The model under review builds one solid part; all positions refer to its coordinate system, in mm. Round coordinates to 2 decimals unless told otherwise and drop trailing zeros. Order: outer loops, then holes, each group sorted by start corner. A loop starts at its lowest first (then second) coordinate and runs counter-clockwise, first axis right, second up.
1) Consider section C-C (y = 0.2). Give the number of separate pieces and of enclosed holes in the cut face, then the cut area to 3 significant figures.
2) Consider section B-B (x = 0). Give the boundary of the cut face in (y, z), then the cut area to 4 significant figures.
3) Consider section D-D (z = 1). Give the boundary of the cut face in (x, y).
4) Consider section A-A (x = 5.1). Give the boundary of the cut face in (y, z).
5) To check wall thickness, follow L1, parallel to X at y = 0.1, z = 5.5; L2, parallel to Z at x = -2.3, y = 0.15; L3, parallel to X at y = 0.25, z = 1.25. State the ranges of each line that lie inside material, in increasing order.
from build123d import *

# Parameters (mm, degrees)
EXTRUDE1_DEPTH = 0.3
SKETCH3_R      = 0.4
SKETCH3_W      = 3
SKETCH3_H      = 1.2
EXTRUDE2_DEPTH = 1.3
SKETCH4_W      = 1
SKETCH4_H      = 0.25
EXTRUDE3_DEPTH = 24
SKETCH5_W      = 1.5
SKETCH5_H      = 1.5
EXTRUDE5_DEPTH = 1


with BuildPart() as part:
    # Sketch1 → Extrude1 (new body)
    with BuildSketch(Plane(origin=(0, 0, 0), x_dir=(1, 0, 0), z_dir=(0, 1, 0))):
        with BuildLine():
            Line((-2.435487214, 9.089362025), (-2.915825654, 7.984232008))
            ThreePointArc((-2.915825654, 7.984232008), (-4.25, 7.361215932), (-5.456634922, 6.517295093))
            Line((-5.456634922, 6.517295093), (-6.653874811, 6.653874811))
            Line((-6.653874811, 6.653874811), (-6.517295093, 5.456634922))
            ThreePointArc((-6.517295093, 5.456634922), (-7.361215932, 4.25), (-7.984232008, 2.915825654))
            Line((-7.984232008, 2.915825654), (-9.089362025, 2.435487214))
            Line((-9.089362025, 2.435487214), (-8.372460576, 1.466936915))
            ThreePointArc((-8.372460576, 1.466936915), (-8.5, 0), (-8.372460576, -1.466936915))
            Line((-8.372460576, -1.466936915), (-9.089362025, -2.435487214))
            Line((-9.089362025, -2.435487214), (-7.984232008, -2.915825654))
            ThreePointArc((-7.984232008, -2.915825654), (-7.361215932, -4.25), (-6.517295093, -5.456634922))
            Line((-6.517295093, -5.456634922), (-6.653874811, -6.653874811))
            Line((-6.653874811, -6.653874811), (-5.456634922, -6.517295093))
            ThreePointArc((-5.456634922, -6.517295093), (-4.25, -7.361215932), (-2.915825654, -7.984232008))
            Line((-2.915825654, -7.984232008), (-2.435487214, -9.089362025))
            Line((-2.435487214, -9.089362025), (-1.466936915, -8.372460576))
            ThreePointArc((-1.466936915, -8.372460576), (0, -8.5), (1.466936915, -8.372460576))
            Line((1.466936915, -8.372460576), (2.435487214, -9.089362025))
            Line((2.435487214, -9.089362025), (2.915825654, -7.984232008))
            ThreePointArc((2.915825654, -7.984232008), (4.25, -7.361215932), (5.456634922, -6.517295093))
            Line((5.456634922, -6.517295093), (6.653874811, -6.653874811))
            Line((6.653874811, -6.653874811), (6.517295093, -5.456634922))
            ThreePointArc((6.517295093, -5.456634922), (7.361215932, -4.25), (7.984232008, -2.915825654))
            Line((7.984232008, -2.915825654), (9.089362025, -2.435487214))
            Line((9.089362025, -2.435487214), (8.372460576, -1.466936915))
            ThreePointArc((8.372460576, -1.466936915), (8.5, 0), (8.372460576, 1.466936915))
            Line((8.372460576, 1.466936915), (9.089362025, 2.435487214))
            Line((9.089362025, 2.435487214), (7.984232008, 2.915825654))
            ThreePointArc((7.984232008, 2.915825654), (7.361215932, 4.25), (6.517295093, 5.456634922))
            Line((6.517295093, 5.456634922), (6.653874811, 6.653874811))
            Line((6.653874811, 6.653874811), (5.456634922, 6.517295093))
            ThreePointArc((5.456634922, 6.517295093), (4.25, 7.361215932), (2.915825654, 7.984232008))
            Line((2.915825654, 7.984232008), (2.435487214, 9.089362025))
            Line((2.435487214, 9.089362025), (1.466936915, 8.372460576))
            ThreePointArc((1.466936915, 8.372460576), (0, 8.5), (-1.466936915, 8.372460576))
            Line((-1.466936915, 8.372460576), (-2.435487214, 9.089362025))
        make_face()
    extrude(amount=EXTRUDE1_DEPTH)

    # Sketch3 → Extrude2 (cut, through all)
    with BuildSketch(Plane(origin=(0, 0, 0), x_dir=(1, 0, 0), z_dir=(0, 1, 0))):
        with Locations((-2.3, 0)):
            Circle(SKETCH3_R)
        with Locations((-3.625, 0)):
            Circle(SKETCH3_R)
        with Locations((-5.1, 0)):
            Circle(SKETCH3_R)
        with Locations((2.3, 0)):
            Circle(SKETCH3_R)
        with Locations((3.625, 0)):
            Circle(SKETCH3_R)
        with Locations((5.1, 0)):
            Circle(SKETCH3_R)
        Rectangle(SKETCH3_W, SKETCH3_H)
    extrude(amount=EXTRUDE2_DEPTH, mode=Mode.SUBTRACT)

    # Sketch4 → Extrude3 (cut)
    with BuildSketch(Plane(origin=(0, 0, 0), x_dir=(1, 0, 0), z_dir=(0, 1, 0))):
        with Locations((0, -1.625)):
            Rectangle(SKETCH4_W, SKETCH4_H)
    extrude(amount=EXTRUDE3_DEPTH, mode=Mode.SUBTRACT)

    # Sketch5 → Extrude5 (cut)
    with BuildSketch(Plane(origin=(0, 0, 0), x_dir=(1, 0, 0), z_dir=(0, 1, 0))):
        with Locations((-8.65, -0.75)):
            Rectangle(SKETCH5_W, SKETCH5_H)
        with Locations((8.65, -0.75)):
            Rectangle(SKETCH5_W, SKETCH5_H)
    extrude(amount=EXTRUDE5_DEPTH, mode=Mode.SUBTRACT)


solid = part.part
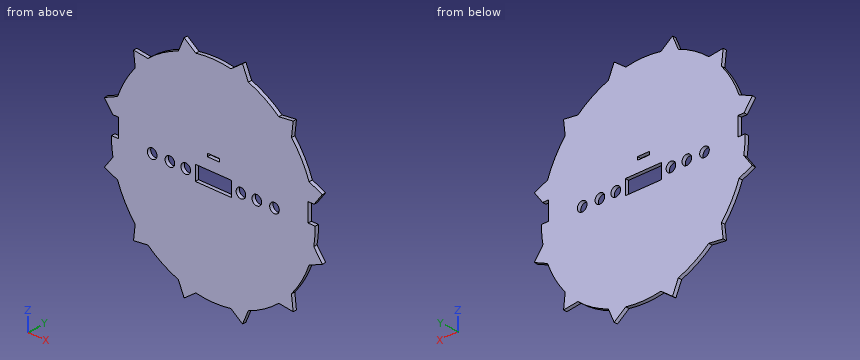
Answer below:
1. separate pieces: 1
1. enclosed holes: 8
1. area: 227 mm2
2. outline: (0, -8.5) - (0.3, -8.5) - (0.3, -0.6) - (0, -0.6) - close; (0, 0.6) - (0.3, 0.6) - (0.3, 1.5) - (0, 1.5) - close; (0, 1.75) - (0.3, 1.75) - (0.3, 8.5) - (0, 8.5) - close
2. area: 4.665 mm2
3. outline: (-7.9, 0) - (7.9, 0) - (7.9, 0.3) - (-7.9, 0.3) - close
4. outline: (0, -6.8) - (0.3, -6.8) - (0.3, -0.4) - (0, -0.4) - close; (0, 0.4) - (0.3, 0.4) - (0.3, 6.8) - (0, 6.8) - close
5. L1: x = -6.52 to 6.52
5. L2: z = -8.99 to -0.4, 0.4 to 8.99
5. L3: x = -7.9 to 7.9
